For this review, take the finished solid that the model builds, in its own axes (mm). A direction names the side the tool comes from. Coordinates: 2 decimals unless noted, no trailing zeros. Loops run counter-clockwise (first coordinate to the right, second up) from the corner with the lowest first, then second, coordinate; pieces in that order, holes last.
```python
from build123d import *
from build123d.topology import SkipClean

# Parameters (mm, degrees)
SKETCH1_R           = 2.1
BOSS_EXTRUDE1_DEPTH = 20
SKETCH3_R           = 2.6
BOSS_EXTRUDE2_DEPTH = 17.5


with BuildPart() as part:
    # Sketch1 → Boss-Extrude1 (new body)
    with BuildSketch(Plane(origin=(0, 0, 0), x_dir=(1, 0, 0), z_dir=(0, 1, 0))):
        with BuildLine():
            Line((-7.75, -12.5), (-7.75, 0))
            Line((-7.75, 0), (-51, 0))
            Line((-51, 0), (-51, -4))
            Line((-51, -4), (-23.75, -4))
            ThreePointArc((-23.75, -4), (-19.507359313, -5.757359313), (-17.75, -10))
            Line((-17.75, -10), (-17.75, -12.5))
            ThreePointArc((-17.75, -12.5), (-12.75, -17.5), (-7.75, -12.5))
        make_face()
        with Locations(Location((-12.75, -12.5, 0), (0, 0, 270))):
            Circle(SKETCH1_R, mode=Mode.SUBTRACT)
    extrude(amount=BOSS_EXTRUDE1_DEPTH)


with BuildPart() as body_2:
    # Sketch3 → Boss-Extrude2 (new, through all)
    with BuildSketch(Plane.XY):
        with BuildLine():
            Line((-51, 0), (-7.75, 0))
            Line((-7.75, 0), (-7.75, 10))
            Line((-7.75, 10), (-17.715728753, 10))
            ThreePointArc((-17.715728753, 10), (-21.542563076, 10.761204675), (-24.786796564, 12.928932188))
            Line((-24.786796564, 12.928932188), (-28.928932188, 17.071067812))
            ThreePointArc((-28.928932188, 17.071067812), (-32.173165676, 19.238795325), (-36, 20))
            Line((-36, 20), (-51, 20))
            Line((-51, 20), (-51, 12.6))
            ThreePointArc((-51, 12.6), (-49.161522369, 11.838477631), (-48.4, 10))
            ThreePointArc((-48.4, 10), (-49.161522369, 8.161522369), (-51, 7.4))
            Line((-51, 7.4), (-51, 0))
        make_face()
        with Locations((-36, 10)):
            Circle(SKETCH3_R, mode=Mode.SUBTRACT)
    extrude(amount=BOSS_EXTRUDE2_DEPTH)

    # Intersect1: read off the stored shape, not the designer's step
    # Intersect1: intersect part
    add(part.part, mode=Mode.INTERSECT)

    # Mirror1: body 2 across face


with BuildPart() as body_2_1:
    with SkipClean():  # the faces are left unmerged after this step: merging them gives an invalid solid
        add(body_2.part)
        add(body_2.part.mirror(Plane(origin=(-51, 16.3, 2), x_dir=(0, 0, 1), z_dir=(-1, 0, 0))))


solid = body_2_1.part
```
Q1. Wall thickness on probe 1 along X at (y, z) = (5.75, 12.5); probe 2 along Z at (x, y) = (-12.75, 3.25); probe 3 along X at (y, z) = (3.75, 6.5): over which ranges is each line inside the solid? List them lowest first.
Q2. Consider section D-D (x = -47.5). State the section outline as (y, z) points.
Q3. The part is to be moulded in two halves that separate along X. For faces 1 (the face through (-63.4, 10.1, 2)), 2 (the face through (-75.17, 14.97, 1.97)), 3 (the face through (-26.83, 14.97, 1.97)), say which applies: +X half, -X half, draft (parallel to the pull), parting line (faces both ways), or undercut.
Q4. For pin 1 Ø5 at (x, y) = (-33.5, 8) entering from +Z; pin 2 Ø5 at (x, z) = (-12.5, 8.5) entering from +Y; pin 3 Ø1.5 at (x, z) = (-25.5, 3) entering from +Y, all flat-tipped, find the tip position at first contact; note any pin that passes through.
Q5. Consider section A-A (z = 5.75). State the section outline as (x, y) points.
Q6. Machinability: for faces 4 (the face through (-17.75, 5, 11)), 5 (the face through (-51, 20, 2)), 6 (the face through (-89, 10, 9)), which of the approach directions +Z, -Z, +X, -X, +Y, -Y give a long, thin tool a straight path to every point of the face, cutting with its end or side? Answer none if there is none.
Q7. Consider section B-B (y = 4.5). State the section outline as (x, z) points, then the cut area to 3 significant figures.
Q8. Consider section C-C (z = 2.5). State the section outline as (x, y) points, then the cut area to 3 significant figures.
Model answer:
1. probe 1: x = -94.25 to -91.35, -87.15 to -84.25, -17.75 to -14.85, -10.65 to -7.75
1. probe 2: z = 0 to 10.4, 14.6 to 17.5
1. probe 3: x = -94.25 to -83.12, -18.88 to -7.75
2. outline: (0, 0) - (20, 0) - (20, 4) - (0, 4) - close
3. face 1: undercut
3. face 2: -X half
3. face 3: +X half
4. pin 1: stops at z = 4
4. pin 2: stops at y = 10
4. pin 3: stops at y = 14.39
5. outline: (-94.25, 0) - (-82.49, 0) - (-82.49, 10.16) arc R10 cw to (-84.28, 10) - (-94.25, 10) - close; (-19.51, 0) - (-7.75, 0) - (-7.75, 10) - (-17.72, 10) arc R10 cw to (-19.51, 10.16) - close
6. face 4: +Z, +Y, -Y
6. face 5: +Z, -Z, +X, -X, +Y
6. face 6: +Z, -Z, -X, +Y
7. outline: (-94.25, 0) - (-7.75, 0) - (-7.75, 12.5) arc R5 ccw to (-17.75, 12.5) - (-17.75, 10) arc R6 cw to (-23.75, 4) - (-78.25, 4) arc R6 cw to (-84.25, 10) - (-84.25, 12.5) arc R5 ccw to (-94.25, 12.5) - close; hole circle Ø4.2 at (-89.25, 12.5); hole circle Ø4.2 at (-12.75, 12.5)
7. area: 582 mm2
8. outline: (-94.25, 0) - (-7.75, 0) - (-7.75, 10) - (-17.72, 10) arc R10 cw to (-24.79, 12.93) - (-28.93, 17.07) arc R10 ccw to (-36, 20) - (-66, 20) arc R10 ccw to (-73.07, 17.07) - (-77.21, 12.93) arc R10 cw to (-84.28, 10) - (-94.25, 10) - close; hole circle Ø5.2 at (-66, 10); hole circle Ø5.2 at (-51, 10); hole circle Ø5.2 at (-36, 10)
8. area: 1,280 mm2
